```python
from build123d import *

# Parameters (mm, degrees)
SKETCH_1_R          = 12.5
EXTRUDE_1_DEPTH     = 65.5
SKETCH_2_R          = 5
EXTRUDE_2_DEPTH     = 4
SKETCH_3_R          = 1.5
EXTRUDE_3_DEPTH     = 12.5
SKETCH_4_R          = 1
CUT_EXTRUDE_1_DEPTH = 10


with BuildPart() as part:
    # 스케치1 → 돌출1 (new body)
    with BuildSketch(Plane.XY):
        Circle(SKETCH_1_R)
    extrude(amount=EXTRUDE_1_DEPTH)

    # 스케치2 → 돌출2 (add)
    with BuildSketch(Plane.XY.offset(65.5)):
        Circle(SKETCH_2_R)
    extrude(amount=EXTRUDE_2_DEPTH)

    # 스케치3 → 돌출3 (add)
    with BuildSketch(Plane.XY.offset(65.5)):
        Circle(SKETCH_3_R)
    extrude(amount=EXTRUDE_3_DEPTH)

    # 스케치4 → 컷-돌출1 (cut)
    with BuildSketch(Plane.XY.offset(65.5)):
        with Locations((0, 8.5)):
            Circle(SKETCH_4_R)
        with Locations((0, -8.5)):
            Circle(SKETCH_4_R)
        with Locations((-7.361215932, -4.25)):
            Circle(SKETCH_4_R)
        with Locations((7.361215932, -4.25)):
            Circle(SKETCH_4_R)
    extrude(amount=-CUT_EXTRUDE_1_DEPTH, mode=Mode.SUBTRACT)


solid = part.part
```
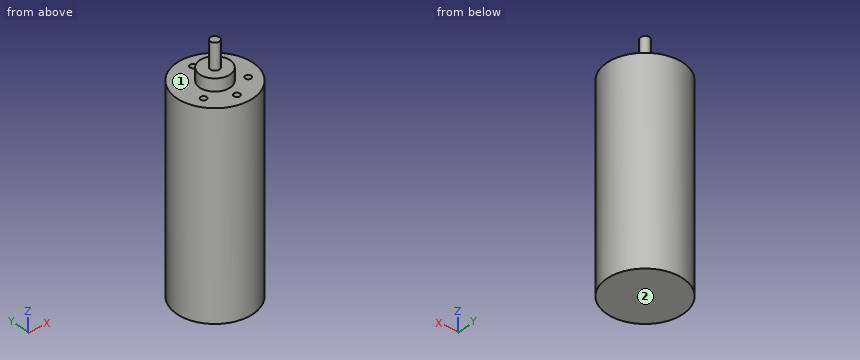
Read the model definition and answer for the solid it produces. Units are mm, in the model's axes. Face numbers are marked on the shaded views. A direction names the side the tool comes from. Give positions to 0.01 mm unless a question says otherwise; leave off trailing zeros. Loops run counter-clockwise (first coordinate to the right, second up) from the corner with the lowest first, then second, coordinate; pieces in that order, holes last.
Item 1: Find the intervals of material crossed by line 1 along Y through (x, z) = (0, 63.5); line 2 along Z through (x, y) = (-4.75, -10.25); line 3 along Z through (x, y) = (-0.5, -2.5), in increasing order.
Item 2: For the marked faces 1 and 2, determine the directions among +Z, -Z, +X, -X, +Y, -Y from which every point of the face is accessible in a straight line to the end or side of a thin tool.
Item 3: The part is cut by section A-A (x = 0). Write down the section's boundary in (y, z), and give its area (3 significant figures).
Item 4: The part is cut by section C-C (z = 72.5). Write down the section's boundary in (x, y), and give its area (3 significant figures).
Item 5: The part is cut by section B-B (y = 3). Write down the section's boundary in (x, z).
Item 6: The part is cut by section D-D (y = -4.25). Write down the section's boundary in (x, z).
Item 7: Each of these flat-tipped pins is pushed along its axis until it touches: pin 1 Ø0.6 at (x, y) = (7, -4) entering from +Z; pin 2 Ø6 at (x, z) = (-3, 67.5) entering from -Y; pin 3 Ø2 at (x, y) = (-0.5, 8) entering from +Z. Where does it stop, or does it pass through?
Taken from the geometry:
1. line 1: y = -12.5 to -9.5, -7.5 to 7.5, 9.5 to 12.5
1. line 2: z = 0 to 65.5
1. line 3: z = 0 to 69.5
2. face 1: +Z
2. face 2: -Z, +X, -X, +Y, -Y
3. outline: (-12.5, 0) - (12.5, 0) - (12.5, 65.5) - (9.5, 65.5) - (9.5, 55.5) - (7.5, 55.5) - (7.5, 65.5) - (5, 65.5) - (5, 69.5) - (1.5, 69.5) - (1.5, 78) - (-1.5, 78) - (-1.5, 69.5) - (-5, 69.5) - (-5, 65.5) - (-7.5, 65.5) - (-7.5, 55.5) - (-9.5, 55.5) - (-9.5, 65.5) - (-12.5, 65.5) - close
3. area: 1,660 mm2
4. outline: circle Ø3 at (0, 0)
4. area: 7.07 mm2
5. outline: (-12.13, 0) - (12.13, 0) - (12.13, 65.5) - (4, 65.5) - (4, 69.5) - (-4, 69.5) - (-4, 65.5) - (-12.13, 65.5) - close
6. outline: (-11.76, 0) - (11.76, 0) - (11.76, 65.5) - (8.36, 65.5) - (8.36, 55.5) - (6.36, 55.5) - (6.36, 65.5) - (2.63, 65.5) - (2.63, 69.5) - (-2.63, 69.5) - (-2.63, 65.5) - (-6.36, 65.5) - (-6.36, 55.5) - (-8.36, 55.5) - (-8.36, 65.5) - (-11.76, 65.5) - close
7. pin 1: stops at z = 55.5
7. pin 2: stops at y = -12.48
7. pin 3: stops at z = 65.5
